Can you work these out from the drawing? Everything is in mm from the part's minimum corner. A direction names the side the tool comes from. Coordinates: 2 decimals unless noted, no trailing zeros. Order: outer loops, then holes, each group sorted by start corner. A loop starts at its lowest first (then second) coordinate and runs counter-clockwise, first axis right, second up. Notation, with made-up numbers: (88.5, 11) -> (109.5, 11) arc R25 cw to (109.5, 50) -> close; hole circle Ø5 at (53.5, -11). An arc over 180 degrees is marked (long way). Put each result on its own line as item: value. Start each with the question number.
Q1. If we section it at B-B (x = 5.75): Please give me the cut outline in (y, z), and give its area (3 significant figures).
Q2. Please list where these lines run through material, in increasing order: line 1 along Z through (x, y) = (8, 7.5); line 2 along Y through (x, z) = (9, 11.25); line 3 along X through (y, z) = (8.75, 16.5).
Q3. If we section it at A-A (z = 14.25): Please give me the cut outline in (x, y) (3 decimals).
Q4. If we section it at C-C (y = 1): Please give me the cut outline in (x, z), and give its area (3 significant figures).
Q5. Will these pins go through, and if not, where does the flat tip stop? pin 1 (4 mm diameter, centred on x = 5, y = 7.5, fed in from +Z); pin 2 (1.5 mm diameter, centred on x = 2.5, z = 21, fed in from -Y); pin 3 (1.5 mm diameter, centred on x = 6, z = 21.5, fed in from -Y); pin 4 (1.5 mm diameter, centred on x = 10.5, z = 15.5, fed in from +Y).
Q6. For the marked faces 1 and 2, which set-ups out of +Z, -Z, +X, -X, +Y, -Y let a thin tool reach every point of the face, with its end or its side?
Q7. If we section it at D-D (x = 3.5): Please give me the cut outline in (y, z), and give its area (3 significant figures).
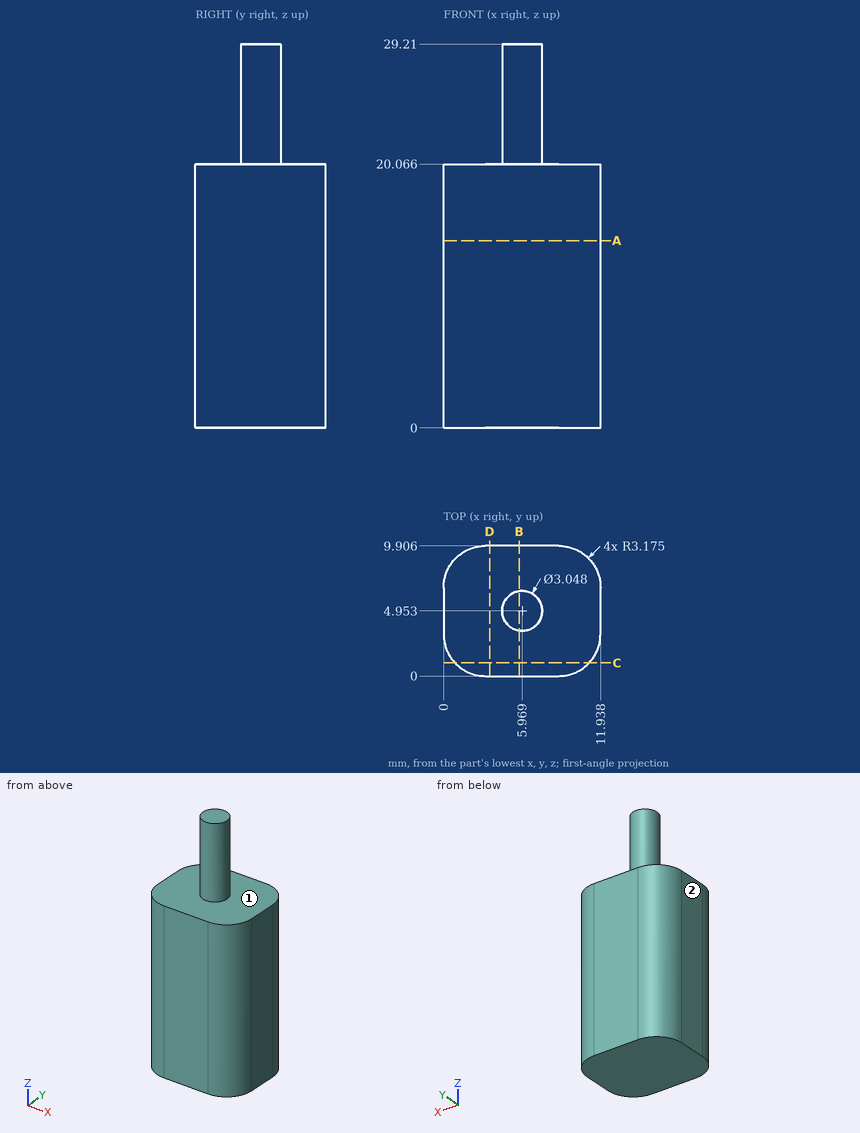
The answers:
1. outline: (0, 0) -> (9.91, 0) -> (9.91, 20.07) -> (6.46, 20.07) -> (6.46, 29.21) -> (3.44, 29.21) -> (3.44, 20.07) -> (0, 20.07) -> close
1. area: 226 mm^2
2. line 1: 0 to 20.07
2. line 2: 0.01 to 9.9
2. line 3: 0.72 to 11.21
3. outline: (0, 3.175) arc R3.175 ccw to (3.175, 0) -> (8.763, 0) arc R3.175 ccw to (11.938, 3.175) -> (11.938, 6.731) arc R3.175 ccw to (8.763, 9.906) -> (3.175, 9.906) arc R3.175 ccw to (0, 6.731) -> close
4. outline: (0.86, 0) -> (11.08, 0) -> (11.08, 20.07) -> (0.86, 20.07) -> close
4. area: 205 mm^2
5. pin 1: z = 29.21
5. pin 2: through
5. pin 3: y = 3.43
5. pin 4: y = 9.75
6. face 1: +Z
6. face 2: +Z, -Z, -X, +Y, -Y
7. outline: (0, 0) -> (9.91, 0) -> (9.91, 20.07) -> (0, 20.07) -> close
7. area: 199 mm^2
